from build123d import *

# Parameters (mm, degrees)
SKETCH1_R           = 50
BOSS_EXTRUDE1_DEPTH = 50
BOSS_EXTRUDE2_REACH = 202
SKETCH2_R           = 45


with BuildPart() as part:
    # Sketch1 → Boss-Extrude1 (new body, symmetric)
    with BuildSketch(Plane.XY):
        with BuildLine():
            Line((-80, -40), (-80, 40))
            Line((-80, 40), (-22.281665693, 61.061668614))
            ThreePointArc((-22.281665693, 61.061668614), (65, 0), (-22.281665693, -61.061668614))
            Line((-22.281665693, -61.061668614), (-80, -40))
        make_face()
        Circle(SKETCH1_R, mode=Mode.SUBTRACT)
    extrude(amount=BOSS_EXTRUDE1_DEPTH, both=True)

    # Sketch2 → Boss-Extrude2 (add, up to next)
    with BuildSketch(Plane(origin=(120, 0, 0), x_dir=(0, 0, -1), z_dir=(1, 0, 0)), mode=Mode.PRIVATE) as boss_extrude2_sk1:
        Circle(SKETCH2_R)
    boss_extrude2_tool1 = extrude(boss_extrude2_sk1.sketch, amount=-BOSS_EXTRUDE2_REACH, mode=Mode.PRIVATE) - part.part
    add(boss_extrude2_tool1.solids().sort_by_distance((120, 0, 0))[0])

    # Sketch5 → Revolve1 (revolve)
    with BuildSketch(Plane.XY):
        Polygon((120, 0), (120, -20), (134, -20), (134, -25), (149, -25), (149, -13.573394096), (157.660254038, -8.573394096), (157.660254038, -3.573394096), (165.660254038, -3.573394096), (175, 0), align=None)
    revolve(axis=Axis((0, 0, 0), (1, 0, 0)))


solid = part.part
Part model, mm, in its own coordinate system. A direction names the side the tool comes from. Give positions to 0.01 mm unless a question says otherwise; leave off trailing zeros. Order: outer loops, then holes, each group sorted by start corner. A loop starts at its lowest first (then second) coordinate and runs counter-clockwise, first axis right, second up. Notation, with made-up numbers: (23, 65.5) - (61, 65.5) arc R26 ccw to (61, 89.5) - close; hole circle Ø10 at (-30.5, -21.75). An arc over 180 degrees is marked (long way). One line per question, with ' | ' between items.
1. Which spindle directions (+Z, -Z, +X, -X, +Y, -Y) get a long thin tool onto all of the face, cutting with end or side? Do faces 1 (the face through (134, -11, -17)), 2 (the face through (-50.737, -50.678, 0.7)), 3 (the face through (149, -11, 11)). Say none if no direction does.
Filled in:
face 1: none | face 2: +Z, -Z, -X, -Y | face 3: +X
2. Band-saw the part on A-A on x = 0. List the corners of the cut face in (y, z), then the cut area to 3 significant figures.
Filled in:
outline: (-65, -50) - (-50, -50) - (-50, 50) - (-65, 50) - close; (50, -50) - (65, -50) - (65, 50) - (50, 50) - close | area: 3,000 mm²
3. Pull direction X, two halves, no side cores. Call faces 4 (the face through (141.605, -23.846, -7.509)), 5 (the face through (-80, -1, 1)), 6 (the face through (47.69, 15.02, -0.7)): +X half, -X half, draft (parallel to the pull), parting line (faces both ways), or undercut.
Filled in:
face 4: draft | face 5: -X half | face 6: undercut
4. Drop flat-ended pins along their axis: P1, Ø12, axis at x = -32.5, z = 31, coming from the +Y side; P2, Ø12, axis at x = 131, z = -10.5, coming from the -Y side; P3, Ø8, axis at x = -51.5, z = 20.5, coming from the +Y side. Give the stop position or say it passes through.
Filled in:
P1: y = 59.52 | P2: y = -24.43 | P3: y = 51.86
5. Drill centre lines: probe 1 along Y at (x, z) = (0, 10); probe 2 along X at (y, z) = (30, -6); probe 3 along X at (y, z) = (-2, 27.5). Where is each one in solid material? Low to high.
Filled in:
probe 1: -65 to -50, 50 to 65 | probe 2: -80 to -40, 40 to 120 | probe 3: -80 to -49.96, 49.96 to 120
6. Band-saw the part on C-C on z = 22.5. List the corners of the cut face in (x, y), then the cut area to 3 significant figures.
Filled in:
outline: (-80, -40) - (-22.28, -61.06) arc R65 ccw to (52.02, -38.97) - (120, -38.97) - (120, 38.97) - (52.02, 38.97) arc R65 ccw to (-22.28, 61.06) - (-80, 40) - close; (134, -10.9) - (149, -10.9) - (149, 10.9) - (134, 10.9) - close; hole circle Ø100 at (0, 0) | area: 12,400 mm²
7. Band-saw the part on D-D on x = 127.5. List the corners of the cut face in (y, z).
Filled in:
outline: circle Ø40 at (0, 0)
8. Band-saw the part on B-B on y = -31.5. List the corners of the cut face in (x, z), then the cut area to 3 significant figures.
Filled in:
outline: (-80, -50) - (-38.83, -50) - (-38.83, 50) - (-80, 50) - close; (38.83, -50) - (56.86, -50) - (56.86, -32.14) - (120, -32.14) - (120, 32.14) - (56.86, 32.14) - (56.86, 50) - (38.83, 50) - close | area: 9,980 mm²
